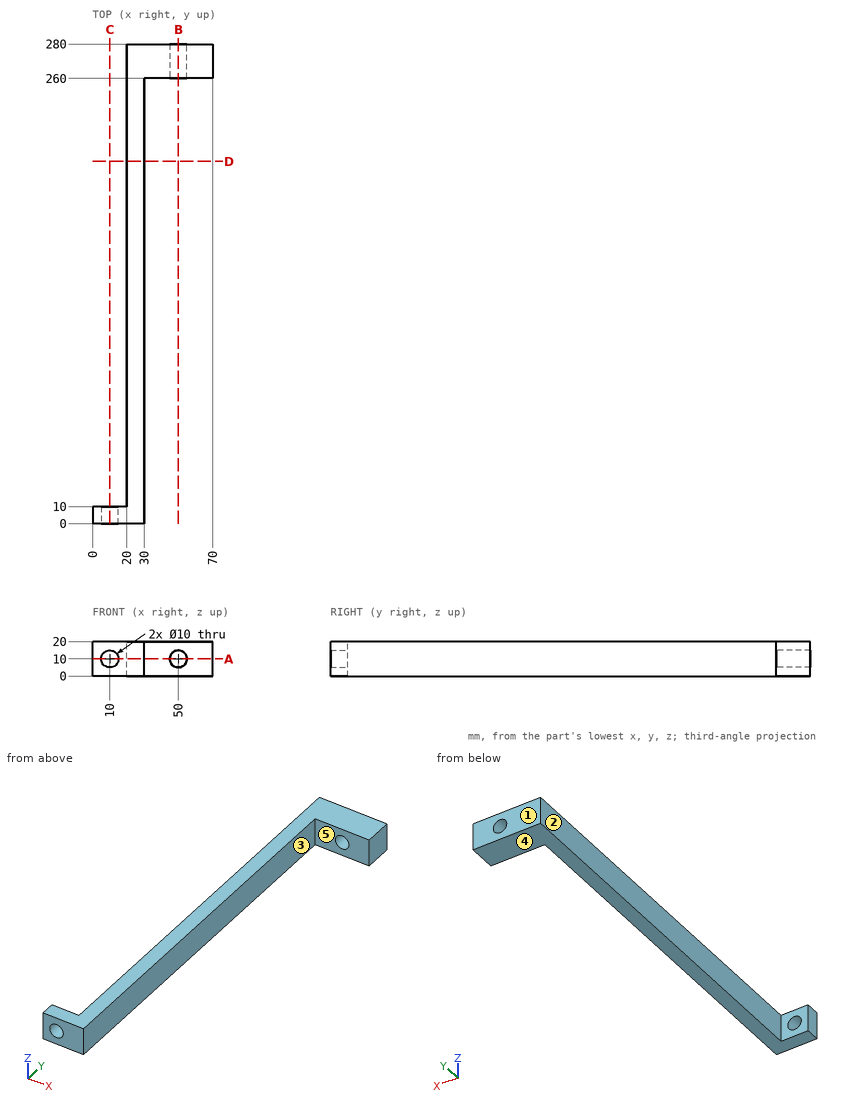
Job drawing, mm, ordinate dimensions from the low corner. One solid piece. A direction names the side the tool comes from. Give positions to 0.01 mm unless a question says otherwise; leave off trailing zeros. Loops run counter-clockwise (first coordinate to the right, second up) from the corner with the lowest first, then second, coordinate; pieces in that order, holes last. Notation, with made-up numbers: M 43.5,82 L 66.5,82 A11 cw 66.5,94 Z; hole C 25,60.25 d9. An arc over 180 degrees is marked long. Use one line per item in the form item = value.
Item 1: Slice it at D-D on y = 211.5. List the corners of the cut face in (x, z), and give its area (3 significant figures).
Filled in:
outline = M 20,0 L 30,0 L 30,20 L 20,20 Z
area = 200 mm^2
Item 2: Which spindle directions (+Z, -Z, +X, -X, +Y, -Y) get a long thin tool onto all of the face, cutting with end or side? Do the marked faces 4 and 5. Say none if no direction does.
Filled in:
face_4 = -Z, +X, -X, +Y, -Y
face_5 = +Z, -Z, +X, -Y
Item 3: Drill centre lines: L1, parallel to Z at x = 10, y = 2; L2, parallel to X at y = 98, z = 7.25; L3, parallel to X at y = 267.5, z = 10. Where is each one in solid material? Low to high.
Filled in:
L1 = 0 to 5, 15 to 20
L2 = 20 to 30
L3 = 20 to 45, 55 to 70
Item 4: Slice it at B-B on x = 50. List the corners of the cut face in (y, z), and give its area (3 significant figures).
Filled in:
outline = M 260,0 L 280,0 L 280,5 L 260,5 Z; M 260,15 L 280,15 L 280,20 L 260,20 Z
area = 200 mm^2
Item 5: Two-plate mould, pull along X, no slides. Class the marked faces 1, 2 and 3: released by +X, released by -X, zero draft, split by the parting line, or undercut.
Filled in:
face_1 = zero draft
face_2 = released by -X
face_3 = released by +X
Item 6: Slice it at A-A on z = 10. List the corners of the cut face in (x, y).
Filled in:
outline = M 0,0 L 5,0 L 5,10 L 0,10 Z; M 15,0 L 30,0 L 30,260 L 45,260 L 45,280 L 20,280 L 20,10 L 15,10 Z; M 55,260 L 70,260 L 70,280 L 55,280 Z
Item 7: Slice it at C-C on x = 10. List the corners of the cut face in (y, z), and give its area (3 significant figures).
Filled in:
outline = M 0,0 L 10,0 L 10,5 L 0,5 Z; M 0,15 L 10,15 L 10,20 L 0,20 Z
area = 100 mm^2
Item 8: Flat gauge pins, fed straight in: pin 1 Ø10 at (y, z) = (106.5, 5.5) entering from +X; pin 2 Ø1.5 at (x, z) = (42.5, 16.5) entering from -Y; pin 3 Ø11.5 at (x, z) = (10, 10) entering from +Y. Where does each tip first touch, or does it go through?
Filled in:
pin_1 = 30
pin_2 = 260
pin_3 = 10
